Here's how the part is built. I have some questions about the finished solid (model axes, mm). Face numbers are marked on the shaded views. A direction names the side the tool comes from. Round coordinates to 2 decimals unless told otherwise and drop trailing zeros. Write each loop counter-clockwise with the first axis right and the second up, starting at its lowest first coordinate (ties: lowest second). Pieces come first, ordered by that corner, then holes. Notation, with made-up numbers: (35.25, 11.5) -> (41.25, 11.5) arc R20 cw to (41.25, 29.5) -> close; hole circle Ø9 at (45.5, -23). An arc over 180 degrees is marked (long way). Put each result on its own line as item: value. Start each with the question number.
1) I want a section at A-A, the plane x = 1.5. List the corners of the cut face in (y, z) for me, then the cut area to 3 significant figures.
2) Which directions (+Z, -Z, +X, -X, +Y, -Y) give clear straight access to the entire face, cutting with the end or side of a thin tool? Please do the marked faces 4, 5, 6 and 7.
3) If I drill on line 1 along X through (y, z) = (1.4, -0.75); line 2 along X through (y, z) = (0.3, -5.5); line 3 along Y through (x, z) = (2.25, -8.75), over which ranges is the centre line in solid material (lowest first)? Write a range as [from, to].
4) We'd pull the mould along Y, two halves only. Please class the marked faces 1, 2 and 3: released by +Y, released by -Y, zero draft, split by the parting line, or undercut.
5) Will these pins go through, and if not, where does the flat tip stop? P1, Ø1.5, axis at x = -1.5, z = -10, coming from the +Y side; P2, Ø0.6, axis at x = -1.5, y = 3.5, coming from the -Z side; P3, Ø0.7, axis at y = 1.5, z = -1, coming from the -X side; P4, Ø1.7, axis at y = 2.5, z = -5, coming from the -X side.
6) I want a section at B-B, the plane z = -6. List the corners of the cut face in (x, y) for me, then the cut area to 3 significant figures.
from build123d import *

# Parameters (mm, degrees)
BOSS_EXTRUDE1_DEPTH = 2
BOSS_EXTRUDE2_DEPTH = 7.4
BOSS_EXTRUDE3_DEPTH = 1.5
FILLET1_R           = 0.5


with BuildPart() as part:
    # Sketch2 → Boss-Extrude1 (new body)
    with BuildSketch(Plane.XY):
        with BuildLine():
            Line((0, 0), (2.78, 0))
            ThreePointArc((2.78, 0), (3.16890873, 0.16109127), (3.33, 0.55))
            Line((3.33, 0.55), (3.33, 1.866025404))
            ThreePointArc((3.33, 1.866025404), (3.347037087, 1.995434926), (3.396987298, 2.116025404))
            Line((3.396987298, 2.116025404), (3.742820323, 2.715025774))
            ThreePointArc((3.742820323, 2.715025774), (3.822740661, 2.907970538), (3.85, 3.115025774))
            Line((3.85, 3.115025774), (3.85, 3.45))
            ThreePointArc((3.85, 3.45), (3.68890873, 3.83890873), (3.3, 4))
            Line((3.3, 4), (0, 4))
            Line((0, 4), (0, 3.7))
            Line((0, 3.7), (3.3, 3.7))
            ThreePointArc((3.3, 3.7), (3.476776695, 3.626776695), (3.55, 3.45))
            Line((3.55, 3.45), (3.55, 3.115025774))
            ThreePointArc((3.55, 3.115025774), (3.532962913, 2.985616251), (3.483012702, 2.865025774))
            Line((3.483012702, 2.865025774), (3.137179677, 2.266025404))
            ThreePointArc((3.137179677, 2.266025404), (3.057259339, 2.07308064), (3.03, 1.866025404))
            Line((3.03, 1.866025404), (3.03, 0.55))
            ThreePointArc((3.03, 0.55), (2.956776695, 0.373223305), (2.78, 0.3))
            Line((2.78, 0.3), (0, 0.3))
            Line((0, 0.3), (0, 0))
        make_face()
    extrude(amount=-BOSS_EXTRUDE1_DEPTH)

    # Sketch4 → Boss-Extrude2 (add)
    with BuildSketch(Plane(origin=(0, 0, -2), x_dir=(-1, 0, 0), z_dir=(0, 0, -1))):
        with BuildLine():
            Line((-3.55, 0), (-3.85, 0))
            Line((-3.85, 0), (-3.85, 3.45))
            ThreePointArc((-3.85, 3.45), (-3.68890873, 3.83890873), (-3.3, 4))
            Line((-3.3, 4), (0, 4))
            Line((0, 4), (0, 3.7))
            Line((0, 3.7), (-3.3, 3.7))
            ThreePointArc((-3.3, 3.7), (-3.476776695, 3.626776695), (-3.55, 3.45))
            Line((-3.55, 3.45), (-3.55, 0))
        make_face()
    extrude(amount=BOSS_EXTRUDE2_DEPTH)

    # Sketch5 → Boss-Extrude3 (add)
    with BuildSketch(Plane(origin=(0, 1.2, 0), x_dir=(1, 0, 0), z_dir=(0, 1, 0))):
        with BuildLine():
            Line((3.85, 9.4), (3.55, 9.4))
            Line((3.55, 9.4), (3.55, 9.6))
            ThreePointArc((3.55, 9.6), (3.619329194, 9.879979456), (3.811294986, 10.095256412))
            Line((3.811294986, 10.095256412), (4.569352507, 10.613690656))
            ThreePointArc((4.569352507, 10.613690656), (4.69484989, 10.805969585), (4.647628206, 11.030671369))
            Line((4.647628206, 11.030671369), (4.221287524, 11.654069155))
            ThreePointArc((4.221287524, 11.654069155), (4.143327639, 11.815508616), (4.116543936, 11.99277417))
            Line((4.116543936, 11.99277417), (4.116543936, 12.4))
            Line((4.116543936, 12.4), (4.416543936, 12.4))
            Line((4.416543936, 12.4), (4.416543936, 11.99277417))
            ThreePointArc((4.416543936, 11.99277417), (4.429935787, 11.904141393), (4.46891573, 11.823421663))
            Line((4.46891573, 11.823421663), (4.895256412, 11.200023877))
            ThreePointArc((4.895256412, 11.200023877), (4.98969978, 10.750620308), (4.738705014, 10.366062451))
            Line((4.738705014, 10.366062451), (3.980647493, 9.847628206))
            ThreePointArc((3.980647493, 9.847628206), (3.884664597, 9.739989728), (3.85, 9.6))
            Line((3.85, 9.6), (3.85, 9.4))
        make_face()
    extrude(amount=BOSS_EXTRUDE3_DEPTH)

    # Fillet1
    fillet1_edges = [part.edges().sort_by_distance(p)[0] for p in [
        (4.266543936, 1.2, -12.4),
        (4.266543936, 2.7, -12.4),
    ]]
    fillet(fillet1_edges, radius=FILLET1_R)

    # Mirror1: part across plane


with BuildPart() as part_1:
    add(part.part)
    add(part.part.mirror(Plane(origin=(0, 4, -2), x_dir=(0, 0, 1), z_dir=(-1, 0, 0))))


solid = part_1.part
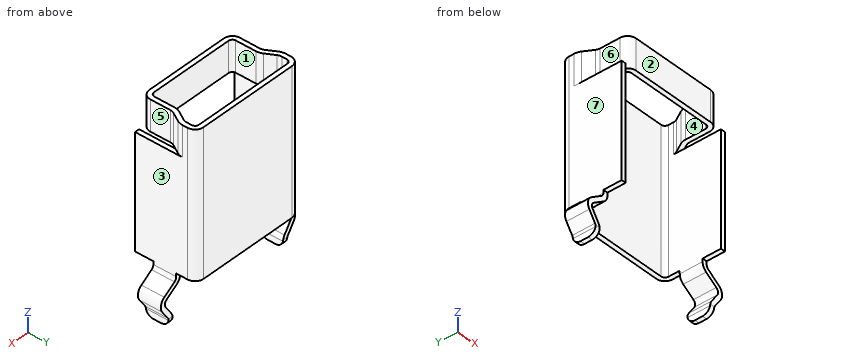
Findings:
1. outline: (0, -2) -> (0.3, -2) -> (0.3, 0) -> (0, 0) -> close; (3.7, -9.4) -> (4, -9.4) -> (4, 0) -> (3.7, 0) -> close
1. area: 3.42 mm2
2. face 4: +Z, -Z
2. face 5: +Z, -Z, +X, -Y
2. face 6: +Z, -Z, -X, -Y
2. face 7: +Z, -X, +Y, -Y
3. line 1: x = [-3.33, -3.03], [3.03, 3.33]
3. line 2: x = [-3.85, -3.55], [3.55, 3.85]
3. line 3: y = [3.7, 4]
4. face 1: undercut
4. face 2: released by -Y
4. face 3: zero draft
5. P1: stops at y = 4
5. P2: stops at z = -9.4
5. P3: stops at x = -3.33
5. P4: stops at x = -3.85
6. outline: (-3.85, 0) -> (-3.55, 0) -> (-3.55, 3.45) arc R0.25 cw to (-3.3, 3.7) -> (3.3, 3.7) arc R0.25 cw to (3.55, 3.45) -> (3.55, 0) -> (3.85, 0) -> (3.85, 3.45) arc R0.55 ccw to (3.3, 4) -> (-3.3, 4) arc R0.55 ccw to (-3.85, 3.45) -> close
6. area: 4.43 mm2
